Part model, mm, in its own coordinate system. Face numbers are marked on the shaded views. Give positions to 0.01 mm unless a question says otherwise; leave off trailing zeros. Write each loop counter-clockwise with the first axis right and the second up, starting at its lowest first coordinate (ties: lowest second). Pieces come first, ordered by that corner, then holes. Notation, with made-up numbers: M 1,8 L 59,8 A19 cw 59,15 Z; hole C 33.5,73 d6. An arc over 180 degrees is marked long. Answer as CSV lines item,"result". Start each with the question number.
1) Slice it at C-C, the plane y = 5. Give the number of separate pieces and of enclosed holes in the cut face, plus the area to 3 significant figures.
2) Mould opens along X. For the marked faces 1, 2 and 3 say: pulls with the +X half, pulls with the -X half, needs draft (parallel to the pull), parting line crosses it, or undercut.
3) Wall check: line 1 along X through (y, z) = (25, -1); line 2 along Y through (x, z) = (5, -1.25); line 3 along Z through (x, y) = (14.25, 25). Give the ranges that are in metal, low to high. Write a range as from..to.
4) Slice it at B-B, the plane z = 1. Give the cut face in (x, y), plus the area to 3 significant figures.
5) Slice it at A-A, the plane x = 5. Give the cut face in (y, z).
6) Pin check, flat tips, straight feed: pin 1 Ø0.6 at (x, y) = (5, 13) entering from +Z; pin 2 Ø0.6 at (x, y) = (11, 12) entering from -Z. Stop position of each tip, or through.
Autodesk Fusion 360 part; units mm, degrees
sketch "Sketch1" plane through (0, 0, 0) normal (0, 0, 1) x (1, 0, 0)
  line L0 (0, 0) -> (25, 0)
  line L1 (25, 0) -> (25, 30)
  line L2 (25, 30) -> (0, 30)
  line L3 (0, 30) -> (0, 0)
  dimension "d1" = 25
  dimension "d2" = 30
extrude "Extrude1" add sketch "Sketch1" along normal blind 4
sketch "Sketch2" plane through (0, 0, 0) normal (0, -1, 0) x (1, 0, 0)
  line L0 (0, 0) -> (25, 0)
  line L1 (25, 0) -> (25, 4)
  line L2 (25, 4) -> (0, 4)
  line L3 (0, 4) -> (0, 0)
  line L4 (25, 2.86) -> (0, 2.86)
  line L5 (0.89, 4) -> (1.1955, 2.86)
  line L6 (2.3645, 2.86) -> (2.67, 4)
  line L7 (3.89, 4) -> (4.1955, 2.86)
  line L8 (5.3645, 2.86) -> (5.67, 4)
  line L9 (6.89, 4) -> (7.1955, 2.86)
  line L10 (8.3645, 2.86) -> (8.67, 4)
  line L11 (9.89, 4) -> (10.1955, 2.86)
  line L12 (11.3645, 2.86) -> (11.67, 4)
  line L13 (12.89, 4) -> (13.1955, 2.86)
  line L14 (14.3645, 2.86) -> (14.67, 4)
  line L15 (15.89, 4) -> (16.1955, 2.86)
  line L16 (17.3645, 2.86) -> (17.67, 4)
  line L17 (18.89, 4) -> (19.1955, 2.86)
  line L18 (20.3645, 2.86) -> (20.67, 4)
  line L19 (21.89, 4) -> (22.1955, 2.86)
  line L20 (23.3645, 2.86) -> (23.67, 4)
  dimension "d5" = 1.14
  dimension "d7" = 1.78
  dimension "d8" = 0.89
  dimension "d11" = 3
  dimension "d12" = 0
  dimension "d15" = 30
extrude "Extrude2" cut sketch "Sketch2" against normal up to surface (30 mm away) contours L2 L4 L5 L6 | L2 L4 L19 L20 | L2 L4 L7 L8 | L2 L4 L17 L18 | L2 L4 L9 L10 | L2 L4 L15 L16 | L2 L4 L11 L12 | L2 L4 L13 L14
sketch "Sketch3" plane through (0, 0, 0) normal (0, 0, -1) x (1, 0, 0)
  line L0 (0, 0) -> (0, -30)
  line L1 (0, -30) -> (25, -30)
  line L2 (25, -30) -> (25, 0)
  line L3 (25, 0) -> (0, 0)
  line L4 (20, -25) -> (5, -25) construction
  line L5 (5, -25) -> (5, -5) construction
  line L6 (5, -5) -> (20, -5) construction
  line L7 (20, -5) -> (20, -25) construction
  circle A0 centre (20, -25) radius 2
  circle A1 centre (5, -25) radius 2
  circle A2 centre (20, -5) radius 2
  circle A3 centre (5, -5) radius 2
  point P0 (12.5, -25)
  point P1 (5, -15)
  point P2 (0, -15)
  point P3 (12.5, -30)
  dimension "d16" = 15
  dimension "d17" = 20
  dimension "d18" = 4
  dimension "d19" = 4
extrude "Extrude3" cut sketch "Sketch3" against normal through all contours A0 | A1 | A2 | A3
mirror "Mirror1" about plane through (0, 0, 0) normal (0, 0, -1) of bodies 1 merged
equation "d8 = ( 1.78 / 2 ) * 1 mm"
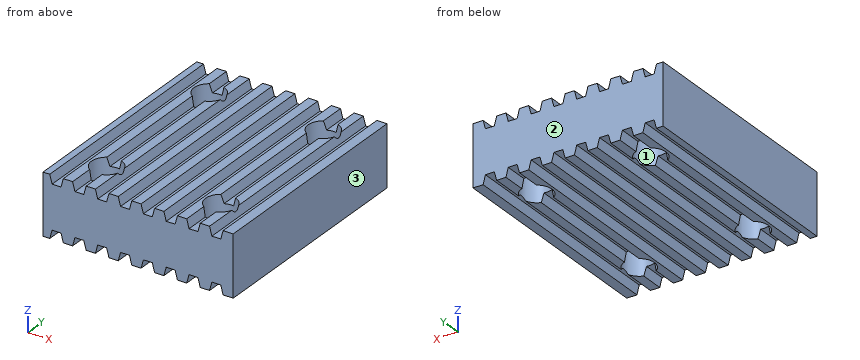
Found:
1,separate pieces,"3"
1,enclosed holes,"0"
1,area,"116 mm²"
2,face 1,"undercut"
2,face 2,"needs draft"
2,face 3,"pulls with the +X half"
3,line 1,"0..3, 7..18, 22..25"
3,line 2,"0..3, 7..23, 27..30"
3,line 3,"-2.86..2.86"
4,outline,"M 0,0 L 25,0 L 25,30 L 0,30 Z; hole C 5,5 d4; hole C 5,25 d4; hole C 20,5 d4; hole C 20,25 d4"
4,area,"700 mm²"
5,outline,"M 0,-2.86 L 3,-2.86 L 3,2.86 L 0,2.86 Z; M 7,-2.86 L 23,-2.86 L 23,2.86 L 7,2.86 Z; M 27,-2.86 L 30,-2.86 L 30,2.86 L 27,2.86 Z"
6,pin 1,"z = 2.86"
6,pin 2,"z = -2.86"
